```python
from build123d import *

# Parameters (mm, degrees)
SKETCH_R        = 1.7
PAD_DEPTH       = 31
SKETCH001_R     = 1.7
POCKET_DEPTH    = 18
CHAMFER_SIZE    = 1
CHAMFER001_SIZE = 1
CHAMFER002_SIZE = 1


with BuildPart() as part:
    # Sketch → Pad (new body)
    with BuildSketch(Plane.XY):
        Polygon((25, 0), (25, 5), (-25, 5), (-25, 0), (-25, -5), (25, -5), align=None)
        with Locations((-20, 0)):
            Circle(SKETCH_R, mode=Mode.SUBTRACT)
        with Locations((20, 0)):
            Circle(SKETCH_R, mode=Mode.SUBTRACT)
    extrude(amount=PAD_DEPTH)

    # Sketch001 (on Face3 of Pad) → Pocket (cut)
    with BuildSketch(Plane.XZ.offset(5)):
        with Locations((0, 23.45)):
            Circle(SKETCH001_R)
        with Locations((0, 7.55)):
            Circle(SKETCH001_R)
    extrude(amount=-POCKET_DEPTH, mode=Mode.SUBTRACT)

    # Chamfer
    chamfer_edges = [part.edges().sort_by_distance(p)[0] for p in [
        (-21.7, 0, 31),
        (18.3, 0, 31),
        (-21.7, 0, 0),
        (18.3, 0, 0),
    ]]
    chamfer(chamfer_edges, length=CHAMFER_SIZE)

    # Chamfer001
    chamfer001_edges = [part.edges().sort_by_distance(p)[0] for p in [
        (-1.7, -5, 23.45),
        (-1.7, -5, 7.55),
        (-1.7, 5, 7.55),
        (-1.7, 5, 23.45),
    ]]
    chamfer(chamfer001_edges, length=CHAMFER001_SIZE)

    # Chamfer002
    chamfer002_edges = [part.edges().sort_by_distance(p)[0] for p in [
        (25, 5, 15.5),
        (25, -5, 15.5),
        (-25, -5, 15.5),
        (-25, 5, 15.5),
        (0, 5, 31),
        (0, -5, 31),
        (-25, 0, 31),
        (25, 0, 31),
        (25, 0, 0),
        (0, -5, 0),
        (0, 5, 0),
        (-25, 0, 0),
    ]]
    chamfer(chamfer002_edges, length=CHAMFER002_SIZE)


solid = part.part
```
Verification items for the finished model (mm, model axes). Give positions to 0.01 mm unless a question says otherwise; leave off trailing zeros. Order: outer loops, then holes, each group sorted by start corner. A loop starts at its lowest first (then second) coordinate and runs counter-clockwise, first axis right, second up. Notation, with made-up numbers: (-1.75, -11) -> (54.25, -11) arc R20 cw to (54.25, 2) -> close; hole circle Ø8 at (-9.75, 77). An arc over 180 degrees is marked (long way). Use a Markdown table: item, result.
1) Section check C-C, the plane x = -20. Record the boundary of the cut face in (y, z), then the cut area to 3 significant figures.
Results:
| item | result |
|---|---|
| outline | (-5, 1) -> (-4, 0) -> (-2.7, 0) -> (-1.7, 1) -> (-1.7, 30) -> (-2.7, 31) -> (-4, 31) -> (-5, 30) -> close; (1.7, 1) -> (2.7, 0) -> (4, 0) -> (5, 1) -> (5, 30) -> (4, 31) -> (2.7, 31) -> (1.7, 30) -> close |
| area | 201 mm² |
2) Depth check by flat-ended pin: pin 1 Ø4 at (x, y) = (-20, 0) entering from +Z; pin 2 Ø4 at (x, z) = (0, 23.45) entering from +Y. Enter the tip coordinate at first touch or a pass-through.
Results:
| item | result |
|---|---|
| pin 1 | z = 30.3 |
| pin 2 | y = 4.3 |
3) Section check A-A, the plane y = 0. Record the boundary of the cut face in (x, z), then the cut area to 3 significant figures.
Results:
| item | result |
|---|---|
| outline | (-25, 1) -> (-24, 0) -> (-22.7, 0) -> (-21.7, 1) -> (-21.7, 30) -> (-22.7, 31) -> (-24, 31) -> (-25, 30) -> close; (-18.3, 1) -> (-17.3, 0) -> (17.3, 0) -> (18.3, 1) -> (18.3, 30) -> (17.3, 31) -> (-17.3, 31) -> (-18.3, 30) -> close; (21.7, 1) -> (22.7, 0) -> (24, 0) -> (25, 1) -> (25, 30) -> (24, 31) -> (22.7, 31) -> (21.7, 30) -> close; hole circle Ø3.4 at (0, 7.55); hole circle Ø3.4 at (0, 23.45) |
| area | 1,320 mm² |
4) Section check B-B, the plane z = 23.45. Record the boundary of the cut face in (x, y).
Results:
| item | result |
|---|---|
| outline | (-25, -4) -> (-24, -5) -> (-2.7, -5) -> (-1.7, -4) -> (-1.7, 4) -> (-2.7, 5) -> (-24, 5) -> (-25, 4) -> close; (1.7, -4) -> (2.7, -5) -> (24, -5) -> (25, -4) -> (25, 4) -> (24, 5) -> (2.7, 5) -> (1.7, 4) -> close; hole circle Ø3.4 at (-20, 0); hole circle Ø3.4 at (20, 0) |
5) Section check D-D, the plane z = 16. Record the boundary of the cut face in (x, y).
Results:
| item | result |
|---|---|
| outline | (-25, -4) -> (-24, -5) -> (24, -5) -> (25, -4) -> (25, 4) -> (24, 5) -> (-24, 5) -> (-25, 4) -> close; hole circle Ø3.4 at (-20, 0); hole circle Ø3.4 at (20, 0) |
6) Mould release check, pull along Z, two halves, no side actions. Record for faces 1 (the flat face through (-0.3, -4.5, 0.5)), 2 (the flat face through (24.3, -4.3, 30.4)), 3 (the cylindrical face through (-0.221, -0.056, 9.236)): pulls with the +Z half, pulls with the -Z half, needs draft (parallel to the pull), parting line crosses it, or undercut.
Results:
| item | result |
|---|---|
| face 1 | pulls with the -Z half |
| face 2 | pulls with the +Z half |
| face 3 | undercut |
7) Material ranges on probe 1 along Z at (x, y) = (0, -0.5); probe 2 along Y at (x, z) = (20, 21.5); probe 3 along X at (y, z) = (0.5, 15), recorded low to high.
Results:
| item | result |
|---|---|
| probe 1 | 0 to 5.85, 9.25 to 21.75, 25.15 to 31 |
| probe 2 | -5 to -1.7, 1.7 to 5 |
| probe 3 | -25 to -21.62, -18.38 to 18.38, 21.62 to 25 |
